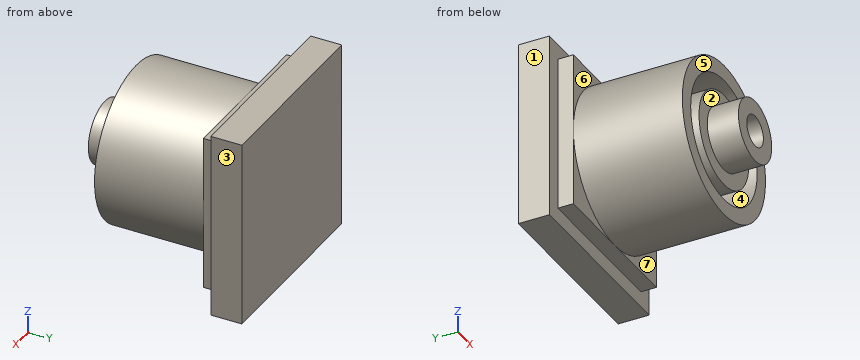
```python
from build123d import *

# Parameters (mm, degrees)
F0_R      = 63.5
F0_R_2    = 38.1
F1_DEPTH  = 12.7
F2_R      = 38.1
F2_R_2    = 25.4
F3_DEPTH  = 127
F4_R      = 25.4
F4_R_2    = 12.7
F5_DEPTH  = 152.4
F6_R      = 63.5
F6_R_2    = 50.8
F7_DEPTH  = 127
F8_W      = 152.4
F8_H      = 152.4
F9_DEPTH  = 25.4
F11_DEPTH = 12.7


with BuildPart() as f1:
    # F0 (on Front) → F1 (new body)
    with BuildSketch(Plane.XZ):
        Circle(F0_R)
        Circle(F0_R_2, mode=Mode.SUBTRACT)
    extrude(amount=F1_DEPTH)

    # F2 (on Front) → F3 (join)
    with BuildSketch(Plane.XZ):
        Circle(F2_R)
        Circle(F2_R_2, mode=Mode.SUBTRACT)
    extrude(amount=F3_DEPTH)

    # F4 (on Front) → F5 (join)
    with BuildSketch(Plane.XZ):
        Circle(F4_R)
        Circle(F4_R_2, mode=Mode.SUBTRACT)
    extrude(amount=F5_DEPTH)

    # F6 (on Front) → F7 (join)
    with BuildSketch(Plane.XZ):
        Circle(F6_R)
        Circle(F6_R_2, mode=Mode.SUBTRACT)
    extrude(amount=F7_DEPTH)

    # F8 (on Front) → F9 (join)
    with BuildSketch(Plane.XZ):
        Rectangle(F8_W, F8_H)
    extrude(amount=F9_DEPTH)

    # F10 (on face) → F11 (join)
    with BuildSketch(Plane.XZ.offset(25.4)):
        with BuildLine():
            Line((1.088e-07, 63.5), (-63.5, 63.5))
            Line((-63.5, 63.5), (-63.5, 0))
            ThreePointArc((-63.5, 0), (-44.9012805669, 44.9012806438), (1.088e-07, 63.5))
        make_face()
        with BuildLine():
            ThreePointArc((-4.16e-08, -63.5), (-44.90128062, -44.9012805906), (-63.5, 0))
            Line((-63.5, 0), (-63.5, -63.5))
            Line((-63.5, -63.5), (-4.16e-08, -63.5))
        make_face()
        with BuildLine():
            Line((63.5, 63.5), (1.088e-07, 63.5))
            ThreePointArc((1.088e-07, 63.5), (44.9012806438, 44.9012805669), (63.5, 0))
            Line((63.5, 0), (63.5, 63.5))
        make_face()
        with BuildLine():
            Line((63.5, -63.5), (63.5, 0))
            ThreePointArc((63.5, 0), (44.9012805906, -44.90128062), (-4.16e-08, -63.5))
            Line((-4.16e-08, -63.5), (63.5, -63.5))
        make_face()
    extrude(amount=F11_DEPTH)


solid = f1.part
```
CAD build for the part. Positions are in the model's coordinates, mm. Face numbers are marked on the shaded views. A direction names the side the tool comes from. Round coordinates to 2 decimals unless told otherwise and drop trailing zeros. Loops run counter-clockwise (first coordinate to the right, second up) from the corner with the lowest first, then second, coordinate; pieces in that order, holes last. Notation, with made-up numbers: (71.5, -21.75) - (116.5, -21.75) arc R27 ccw to (116.5, -3.75) - close; hole circle Ø11 at (17.25, -33). An arc over 180 degrees is marked (long way). Return JSON: item names as keys, results as strings. Group by question number.
Q1. Band-saw the part on D-D on y = -99.5. Give the cut face in (x, z).
Q2. Drill centre lines: line 1 along Z through (x, y) = (0, -59.5); line 2 along X through (y, z) = (-101, -10.5). Where is each one in solid material? Low to high. Write a range as [from, to].
Q3. Band-saw the part on C-C on z = 9. Give the cut face in (x, y).
Q4. Band-saw the part on A-A on y = -31. Give the cut face in (x, z).
Q5. Flat gauge pins, fed straight in: pin 1 Ø2 at (x, y) = (-56.5, -89) entering from +Z; pin 2 Ø14 at (x, y) = (21, -32) entering from -Z; pin 3 Ø6.5 at (y, z) = (-34, -7) entering from +X; pin 4 Ø5 at (x, y) = (-23.5, -126.5) entering from +Z. Where does each tip first touch, or does it go through?
Q6. Tool access for the marked faces 5, 6 and 7: list every direction of +Z, -Z, +X, -X, +Y, -Y with a clear straight run to the whole face (end or side of a thin tool).
Q7. Two-plate mould, pull along X, no slides. Class the marked faces 1, 2, 3 and 4: +X half, -X half, draft (parallel to the pull), parting line (faces both ways), or undercut.
Q8. Band-saw the part on B-B on x = 43.5. Give the cut face in (y, z).
Solutions:
{
 "1": {"outline": "circle Ø127 at (0, 0); circle Ø76.2 at (0, 0); hole circle Ø101.6 at (0, 0); hole circle Ø25.4 at (0, 0)"},
 "2": {"line 1": "z = [-63.5, -50.8], [-38.1, -12.7], [12.7, 38.1], [50.8, 63.5]", "line 2": "x = [-62.63, -49.7], [-36.62, -7.14], [7.14, 36.62], [49.7, 62.63]"},
 "3": {"outline": "(-76.2, -25.4) - (-63.5, -25.4) - (-63.5, -38.1) - (-62.86, -38.1) - (-62.86, -127) - (-50, -127) - (-50, -25.4) - (-37.02, -25.4) - (-37.02, -127) - (-23.75, -127) - (-23.75, -152.4) - (-8.96, -152.4) - (-8.96, -25.4) - (8.96, -25.4) - (8.96, -152.4) - (23.75, -152.4) - (23.75, -127) - (37.02, -127) - (37.02, -25.4) - (50, -25.4) - (50, -127) - (62.86, -127) - (62.86, -38.1) - (63.5, -38.1) - (63.5, -25.4) - (76.2, -25.4) - (76.2, 0) - (-76.2, 0) - close"},
 "4": {"outline": "(-63.5, -63.5) - (63.5, -63.5) - (63.5, 63.5) - (-63.5, 63.5) - close; circle Ø76.2 at (0, 0); hole circle Ø101.6 at (0, 0); hole circle Ø25.4 at (0, 0)"},
 "5": {"pin 1": "stops at z = 30.85", "pin 2": "stops at z = -76.2", "pin 3": "stops at x = 63.5", "pin 4": "stops at z = 59.93"},
 "6": {"face 5": "-Y", "face 6": "+Z, -X, -Y", "face 7": "-Z, +X, -Y"},
 "7": {"face 1": "-X half", "face 2": "draft", "face 3": "+X half", "face 4": "undercut"},
 "8": {"outline": "(-127, -46.26) - (-38.1, -46.26) - (-38.1, -63.5) - (-25.4, -63.5) - (-25.4, -76.2) - (0, -76.2) - (0, 76.2) - (-25.4, 76.2) - (-25.4, 63.5) - (-38.1, 63.5) - (-38.1, 46.26) - (-127, 46.26) - (-127, 26.24) - (-25.4, 26.24) - (-25.4, -26.24) - (-127, -26.24) - close"}
}
